Can you work these out from the model? Positions are in its coordinate system, mm. A direction names the side the tool comes from. Coordinates: 2 decimals unless noted, no trailing zeros. Write each loop counter-clockwise with the first axis right and the second up, starting at its lowest first coordinate (ties: lowest second). Pieces come first, ordered by that corner, then holes. Notation, with made-up numbers: (64.25, 27) - (119.25, 27) arc R16 ccw to (119.25, 37) - close; hole circle Ø10 at (-8.5, 63). An arc over 180 degrees is marked (long way). Write each question's results on one line, items separated by ' | '. Start each with the question number.
```python
from build123d import *

# Parameters (mm, degrees)
BOSS_EXTRUDE1_DEPTH = 3
REVOLVE3_ANGLE      = 20


with BuildPart() as part:
    # Sketch2 → Revolve1 (revolve)
    with BuildSketch(Plane(origin=(0, 0, 0), x_dir=(0, 0, -1), z_dir=(1, 0, 0))):
        with BuildLine():
            Line((45.5, -47.702841719), (45, 0))
            Line((45, 0), (48, 0))
            Line((48, 0), (48.5, -47.702841719))
            ThreePointArc((48.5, -47.702841719), (55.331762509, -68.172170296), (53.883673101, -89.702832813))
            Line((53.883673101, -89.702832813), (51.12598641, -88.963912891))
            ThreePointArc((51.12598641, -88.963912891), (52.533458966, -67.757912773), (45.5, -47.702841719))
        make_face()
    revolve(axis=Axis((0, 50.355486862, 0), (0, -1, 0)))

    # Sketch3 → Revolve2 (revolve)
    with BuildSketch(Plane(origin=(0, 0, 0), x_dir=(0, 0, -1), z_dir=(1, 0, 0))):
        with BuildLine():
            Line((55.784483274, -75.26474612), (60.703757272, -75.26474612))
            Line((60.703757272, -75.26474612), (60.703757272, -78.26474612))
            Line((60.703757272, -78.26474612), (55.703757272, -78.26474612))
            ThreePointArc((55.703757272, -78.26474612), (55.764298122, -76.765289079), (55.784483274, -75.26474612))
        make_face()
    revolve(axis=Axis((0, -123.209470333, 0), (0, 1, 0)))

    # Sketch4 → Boss-Extrude1 (add)
    with BuildSketch(Plane(origin=(0, -75.26474612, 0), x_dir=(1, 0, 0), z_dir=(0, 1, 0))):
        with BuildLine():
            Line((70, 3.743582594), (70, -3.743582594))
            Line((70, -3.743582594), (60.146968721, -8.20294463))
            ThreePointArc((60.146968721, -8.20294463), (60.703757272, 0), (60.146968721, 8.20294463))
            Line((60.146968721, 8.20294463), (70, 3.743582594))
        make_face()
        with BuildLine():
            Line((-70, -3.743582594), (-60.146968721, -8.20294463))
            ThreePointArc((-60.146968721, -8.20294463), (-60.703757272, 0), (-60.146968721, 8.20294463))
            Line((-60.146968721, 8.20294463), (-70, 3.743582594))
            Line((-70, 3.743582594), (-70, -3.743582594))
        make_face()
    extrude(amount=-BOSS_EXTRUDE1_DEPTH)

    # Sketch5 → Revolve3 (revolve, symmetric)
    with BuildSketch(Plane.XY) as revolve3_sk:
        with BuildLine():
            ThreePointArc((51.641833573, -54.16902145), (53.482411948, -55.474645579), (52.935037783, -57.66388395))
            ThreePointArc((52.935037783, -57.66388395), (52.3176263, -55.905651292), (51.641833573, -54.16902145))
        make_face()
        with BuildLine():
            ThreePointArc((54.441970224, -63.100024488), (55.985518381, -64.683651003), (55.126394669, -66.721375297))
            ThreePointArc((55.126394669, -66.721375297), (54.814096651, -64.905046197), (54.441970224, -63.100024488))
        make_face()
    revolve3 = revolve(axis=Axis((0, -123.209470333, 0), (0, 1, 0)), revolution_arc=REVOLVE3_ANGLE / 2)
    revolve3 = revolve3 + revolve(revolve3_sk.sketch, axis=Axis((0, -123.209470333, 0), (0, -1, 0)), revolution_arc=REVOLVE3_ANGLE / 2)

    # Mirror1: Revolve3 across plane
    add(revolve3.mirror(Plane(origin=(0, 0, 0), x_dir=(0, 0, 1), z_dir=(1, 0, 0))))


solid = part.part
```
Q1. Thinking about a two-plate mould opening in Z: for faces 1 (the face through (-1.22, -76.79, 60.69)), 2 (the face through (1.22, -76.79, -60.69)), 3 (the face through (-44.17, -23.52, 9.81)), which applies, pulls with the +Z half, pulls with the -Z half, needs draft (parallel to the pull), parting line crosses it, or undercut?
Q2. I need wall thicknesses on line 1 along Z through (x, y) = (-27.5, -58.5); line 2 along Z through (x, y) = (45, -77); line 3 along Y through (x, z) = (61, 4.5). Which ranges of each line are inside material? Lowest first, please. Write a range as from..to.
Q3. If we section it at B-B (y = -43): Please give me the cut outline in (x, z).
Q4. For faces 4 (the face through (-42.809, -24.185, -22.266)), 5 (the face through (-65.142, -76.744, 5.942)), 6 (the face through (46.34, -78.265, -31.19)), which set-ups out of +Z, -Z, +X, -X, +Y, -Y let a thin tool reach every point of the face, with its end or its side?
Q5. If we section it at A-A (y = -31.5): Please give me the cut outline in (x, z).
Q6. I'm going to push flat-ended pins straight in: pin 1 Ø2 at (x, z) = (44, -28.5) entering from +Y; pin 2 Ø4 at (x, z) = (-35, 22) entering from -Y; pin 3 Ø3 at (y, z) = (-27, 14) entering from +X; pin 4 Ø5 at (x, z) = (13, 47.5) entering from -Y. Where does each tip first touch, or does it pass through?
Answer list:
1) face 1: pulls with the +Z half | face 2: pulls with the -Z half | face 3: undercut
2) line 1: z = -45.55..-42.25, 42.25..45.55 | line 2: z = -40.74..-27.96, 27.96..40.74 | line 3: y = -78.26..-75.26
3) outline: circle Ø96.9 at (0, 0); hole circle Ø90.9 at (0, 0)
4) face 4: +Y | face 5: +Z, -X, +Y, -Y | face 6: -Y
5) outline: circle Ø96.66 at (0, 0); hole circle Ø90.66 at (0, 0)
6) pin 1: stops at y = -53.64 | pin 2: passes through | pin 3: stops at x = 46.64 | pin 4: stops at y = -89.13
